CAD build for the part. Positions are in the model's coordinates, mm. A direction names the side the tool comes from. Give positions to 0.01 mm unless a question says otherwise; leave off trailing zeros. Loops run counter-clockwise (first coordinate to the right, second up) from the corner with the lowest first, then second, coordinate; pieces in that order, holes last.
Item 1: Mould opens along Z. For faces 1 (the cylindrical face through (6.287, -0.078, 10.116)), 2 (the cylindrical face through (18.21, 1.54, 3.13)), 3 (the cylindrical face through (-21.95, 0.01, 5.4)) say: released by +Z, released by -Z, zero draft, split by the parting line, or undercut.
Item 2: Saw through at B-B on z = -1.75. Give the cut face in (x, y), plus the area to 3 significant figures.
Item 3: Probe probe 1 along Z at (x, y) = (-0.5, -15); probe 2 along X at (y, z) = (-4, 9.5); probe 3 along X at (y, z) = (6, 4.5). List the from-to ranges inside material, lowest first.
Item 4: Saw through at A-A on x = 0. Give the cut face in (y, z), plus the area to 3 significant figures.
Item 5: Which spindle directions (+Z, -Z, +X, -X, +Y, -Y) get a long thin tool onto all of the face, cutting with end or side? Do faces 4 (the cylindrical face through (-0.64, 4.91, 9.48)), 5 (the flat face through (20, 0.794, -2)), 6 (the flat face through (-16.51, 0, -2)), 7 (the flat face through (-4, 0, 4.762)). Say none if no direction does.
Item 6: Drop flat-ended pins along their axis: P1, Ø11, axis at x = -2, y = 1.5, coming from the +Z side; P2, Ø4, axis at x = -12, y = 8.5, coming from the -Z side; P3, Ø4, axis at y = -0.5, z = 9, coming from the +X side; P4, Ø1, axis at x = -9, z = 9.5, coming from the +Y side. Give the stop position or say it passes through.
Item 7: Saw through at D-D on y = -8.5. Give the cut face in (x, z), plus the area to 3 significant figures.
from build123d import *

# Parameters (mm, degrees)
F0_R      = 17.4625
F1_DEPTH  = 6.35
F2_R      = 16.51
F3_DEPTH  = 4.7625
F4_R      = 3.81
F5_DEPTH  = 6.351
F6_W      = 6.35
F6_H      = 13.462
F7_DEPTH  = 0.79375
F9_R      = 3.17499
F10_R     = 3.175
F11_R     = 1.651
F12_DEPTH = 18.25725
F13_R     = 6.5405
F13_R_2   = 4.953
F14_DEPTH = 6.35
F16_R     = 1.905
F17_DEPTH = 1.3630747169
F18_R     = 0.59563
F19_DEPTH = 2.7039446902


# Not quite as in the source:
# - a fillet or chamfer is up to 0.001 mm smaller than in the source, because OpenCascade refuses the exact size


with BuildPart() as f1:
    # F0 (on Top) → F1 (new body)
    with BuildSketch(Plane.XY):
        Circle(F0_R)
    extrude(amount=F1_DEPTH)

    # F2 (on face) → F3 (cut)
    with BuildSketch(Plane(origin=(0, 0, 0), x_dir=(1, 0, 0), z_dir=(0, 0, -1))):
        Circle(F2_R)
    extrude(amount=-F3_DEPTH, mode=Mode.SUBTRACT)

    # F4 (on face) → F5 (cut, through all)
    with BuildSketch(Plane.XY.offset(6.35)):
        Circle(F4_R)
    extrude(amount=-F5_DEPTH, mode=Mode.SUBTRACT)

    # F6 (on Front) → F7 (join, symmetric)
    with BuildSketch(Plane.XZ):
        with Locations((-19.685, -0.381)):
            Rectangle(F6_W, F6_H)
    extrude(amount=F7_DEPTH, both=True)

    # F8: F1 across plane


with BuildPart() as f1_1:
    add(f1.part)
    add(f1.part.mirror(Plane.YZ))

    # F9 (radius 3.175 in the source; OpenCascade refuses exactly that, so slightly less here)
    f9_edges = [f1_1.edges().sort_by_distance(p)[0] for p in [
        (-22.86, 0, 6.35),
        (-22.86, 0, -7.112),
        (-16.51, 0, -7.112),
        (22.86, 0, 6.35),
        (22.86, 0, -7.112),
        (16.51, 0, -7.112),
    ]]
    fillet(f9_edges, radius=F9_R)

    # F10 (call 1 of 4: OpenCascade refuses the feature's edges together)
    f10_edges = [f1_1.edges().sort_by_distance(p)[0] for p in [
        (-17.444451, -0.79375, 3.175),
    ]]
    fillet(f10_edges, radius=F10_R)

    # F10#2 (call 2 of 4)
    f10_2_edges = [f1_1.edges().sort_by_distance(p)[0] for p in [
        (-17.444451, 0.79375, 3.175),
    ]]
    fillet(f10_2_edges, radius=F10_R)

    # F10#3 (call 3 of 4)
    f10_3_edges = [f1_1.edges().sort_by_distance(p)[0] for p in [
        (17.444451, -0.79375, 3.175),
    ]]
    fillet(f10_3_edges, radius=F10_R)

    # F10#4 (call 4 of 4)
    f10_4_edges = [f1_1.edges().sort_by_distance(p)[0] for p in [
        (17.444451, 0.79375, 3.175),
    ]]
    fillet(f10_4_edges, radius=F10_R)

    # F11 (on face) → F12 (cut, through all)
    with BuildSketch(Plane(origin=(0, 0.79375, 0), x_dir=(-1, 0, 0), z_dir=(0, 1, 0))):
        with Locations((19.685, -3.937)):
            Circle(F11_R)
        with Locations((-19.685, -3.937)):
            Circle(F11_R)
    extrude(amount=-F12_DEPTH, mode=Mode.SUBTRACT)

    # F13 (on face) → F14 (join)
    with BuildSketch(Plane.XY.offset(6.35)):
        Circle(F13_R)
        Circle(F13_R_2, mode=Mode.SUBTRACT)
    extrude(amount=F14_DEPTH)

    # F16 (on offset) → F17 (join, through all)
    with BuildSketch(Plane.YZ.offset(7.62)):
        with Locations((0, 9.525)):
            Circle(F16_R)
    extrude(amount=-F17_DEPTH)

    # F18 (on face) → F19 (cut, through all)
    with BuildSketch(Plane.YZ.offset(7.62)):
        with Locations((0, 9.525)):
            Circle(F18_R)
    extrude(amount=-F19_DEPTH, mode=Mode.SUBTRACT)


solid = f1_1.part
Results below:
1. face 1: undercut
1. face 2: zero draft
1. face 3: released by +Z
2. outline: (-22.86, -0.79) - (-16.51, -0.79) - (-16.51, 0.79) - (-22.86, 0.79) - close; (16.51, -0.79) - (22.86, -0.79) - (22.86, 0.79) - (16.51, 0.79) - close
2. area: 20.2 mm2
3. probe 1: z = 4.76 to 6.35
3. probe 2: x = -5.17 to -2.92, 2.92 to 5.17
3. probe 3: x = -16.4 to -15.38, 15.38 to 16.4
4. outline: (-17.46, 0) - (-16.51, 0) - (-16.51, 4.76) - (-3.81, 4.76) - (-3.81, 6.35) - (-4.95, 6.35) - (-4.95, 12.7) - (-6.54, 12.7) - (-6.54, 6.35) - (-17.46, 6.35) - close; (3.81, 4.76) - (16.51, 4.76) - (16.51, 0) - (17.46, 0) - (17.46, 6.35) - (6.54, 6.35) - (6.54, 12.7) - (4.95, 12.7) - (4.95, 6.35) - (3.81, 6.35) - close
4. area: 72.6 mm2
5. face 4: +Z
5. face 5: -Z, +X, +Y
5. face 6: -Z, +Y, -Y
5. face 7: -Z
6. P1: stops at z = 12.7
6. P2: stops at z = 0
6. P3: stops at x = 7.62
6. P4: passes through
7. outline: (-15.25, 0) - (-14.15, 0) - (-14.15, 4.76) - (14.15, 4.76) - (14.15, 0) - (15.25, 0) - (15.25, 6.35) - (-15.25, 6.35) - close
7. area: 58.9 mm2
